Source: CAD feature listing. Evaluate the final solid. Frame: model axes, mm. A direction names the side the tool comes from. Give positions to 0.01 mm unless a question says otherwise; leave off trailing zeros. Order: outer loops, then holes, each group sorted by start corner. A loop starts at its lowest first (then second) coordinate and runs counter-clockwise, first axis right, second up. Notation, with made-up numbers: M 7.5,36.5 L 49.5,36.5 A23 cw 49.5,64.5 Z; hole C 60.5,36.25 d1. An arc over 180 degrees is marked long. Use CSV: the item, a comma, the result in double quotes. Start each with the question number.
1. Pin query (flat end, axial travel): P1, Ø3, axis at x = 0, z = 0, coming from the -Y side; P2, Ø5, axis at x = 3, y = 12, coming from the -Z side. Return the tip coordinate at first contact, or that it passes through.
2. Reachability of faces 1 (the flat face through (0, 0, 0)), 2 (the flat face through (-2.5, 21, 2.3)) from +Z, -Z, +X, -X, +Y, -Y: full face, straight path, thin tool, end or side. Return the list, or none.
3. Section query A-A, the plane x = 1. Return the cut outline in (y, z), plus the area to 3 significant figures.
4. Section query D-D, the plane y = 5. Return the cut outline in (x, z), plus the area to 3 significant figures.
5. Section query C-C, the plane z = 2.5. Return the cut outline in (x, y), plus the area to 3 significant figures.
6. Section query B-B, the plane y = 21.25. Return the cut outline in (x, z).
7. Line query: line 1 along Y through (x, z) = (-1, -4.25); line 2 along X through (y, z) = (11.25, -1.75); line 3 along X through (y, z) = (21.5, 2). Output: solid intervals per line, ascending. Write a range as [from, to].
from build123d import *

# Parameters (mm, degrees)
F0_R     = 5
F1_DEPTH = 25
F2_R     = 5
F2_R_2   = 3
F3_DEPTH = 21
F5_DEPTH = 4


with BuildPart() as f1:
    # F0 (on Front) → F1 (new body)
    with BuildSketch(Plane.XZ):
        Circle(F0_R)
    extrude(amount=-F1_DEPTH)

    # F2 (on face) → F3 (cut)
    with BuildSketch(Plane.XZ):
        Circle(F2_R)
        Circle(F2_R_2, mode=Mode.SUBTRACT)
    extrude(amount=-F3_DEPTH, mode=Mode.SUBTRACT)

    # F4 (on face) → F5 (join)
    with BuildSketch(Plane(origin=(0, 25, 0), x_dir=(-1, 0, 0), z_dir=(0, 1, 0))):
        Polygon((2.936192, -4.971128), (5.773219, 0.057253), (2.837027, 5.028381), (-2.936192, 4.971128), (-5.773219, -0.057253), (-2.837027, -5.028381), align=None)
    extrude(amount=-F5_DEPTH)


solid = f1.part
Result set:
1,P1,"y = 0"
1,P2,"z = -2.96"
2,face 1,"+Z, -Z, +X, -X, -Y"
2,face 2,"-Y"
3,outline,"M 0,-2.83 L 21,-2.83 L 21,-5.01 L 25,-5.01 L 25,4.99 L 21,4.99 L 21,2.83 L 0,2.83 Z"
3,area,"159 mm2"
4,outline,"C 0,0 d6"
4,area,"28.3 mm2"
5,outline,"M -4.33,21 L -1.66,21 L -1.66,0 L 1.66,0 L 1.66,21 L 4.33,21 L 4.33,25 L -4.33,25 Z"
5,area,"104 mm2"
6,outline,"M -5.77,0.06 L -2.94,-4.97 L 2.84,-5.03 L 5.77,-0.06 L 2.94,4.97 L -2.84,5.03 Z"
7,line 1,"[21, 25]"
7,line 2,"[-2.44, 2.44]"
7,line 3,"[-4.63, 4.61]"
